Read the model definition and answer for the solid it produces. Units are mm, in the model's axes. A direction names the side the tool comes from. Coordinates: 2 decimals unless noted, no trailing zeros. Order: outer loops, then holes, each group sorted by start corner. A loop starts at its lowest first (then second) coordinate and runs counter-clockwise, first axis right, second up. Notation, with made-up numbers: (-25, -16) -> (-13, -16) arc R20 ccw to (-13, 3) -> close; hole circle Ø10 at (87.25, 28). An arc over 180 degrees is marked (long way). Use CSV: the item, a comma, the result in double quotes.
```python
from build123d import *

# Parameters (mm, degrees)
F1_DEPTH = 80
F2_R     = 7.5
F3_DEPTH = 40
F4_R     = 2.5
F5_DEPTH = 50


with BuildPart() as f1:
    # F0 (on Front) → F1 (new body)
    with BuildSketch(Plane.XZ):
        Polygon((13.916367, 60.022387), (-11.083633, 60.022387), (-11.083633, -19.977613), (-6.383633, -19.977613), (-6.383633, 40.022387), (9.216367, 40.022387), (9.216367, -19.977613), (13.916367, -19.977613), align=None)
    extrude(amount=F1_DEPTH)

    # F2 (on face) → F3 (join)
    with BuildSketch(Plane.XY.offset(60.022387)):
        with Locations((1.416367, -40)):
            Circle(F2_R)
    extrude(amount=F3_DEPTH)

    # F4 (on face) → F5 (cut)
    with BuildSketch(Plane.YZ.offset(13.916367)):
        with Locations((-62.5, -2.477613)):
            Circle(F4_R)
        with Locations((-17.5, -2.477613)):
            Circle(F4_R)
    extrude(amount=-F5_DEPTH, mode=Mode.SUBTRACT)


solid = f1.part
```
Item 1: Find section D-D, the plane x = 11. Give the vertices of the cut face in (y, z).
Return value:
outline,"(-80, -19.98) -> (0, -19.98) -> (0, 60.02) -> (-80, 60.02) -> close; hole circle Ø5 at (-62.5, -2.48); hole circle Ø5 at (-17.5, -2.48)"
Item 2: Find section C-C, the plane y = -40. Give the vertices of the cut face in (x, z).
Return value:
outline,"(-11.08, -19.98) -> (-6.38, -19.98) -> (-6.38, 40.02) -> (9.22, 40.02) -> (9.22, -19.98) -> (13.92, -19.98) -> (13.92, 60.02) -> (8.92, 60.02) -> (8.92, 100.02) -> (-6.08, 100.02) -> (-6.08, 60.02) -> (-11.08, 60.02) -> close"
Item 3: The mould has two halves that part along Y. Classify faces 1 (the flat face through (9.216, -39, 10)), 2 (the cylindrical face through (-0.21, -47.32, 79.74)), 3 (the cylindrical face through (-8.7, -20, -2.4)): +Y half, -Y half, draft (parallel to the pull), parting line (faces both ways), or undercut.
Return value:
face 1,"draft"
face 2,"parting line"
face 3,"undercut"
Item 4: Find section B-B, the plane y = -62.5. Give the vertices of the cut face in (x, z).
Return value:
outline,"(-11.08, -19.98) -> (-6.38, -19.98) -> (-6.38, -4.98) -> (-11.08, -4.98) -> close; (-11.08, 0.02) -> (-6.38, 0.02) -> (-6.38, 40.02) -> (9.22, 40.02) -> (9.22, 0.02) -> (13.92, 0.02) -> (13.92, 60.02) -> (-11.08, 60.02) -> close; (9.22, -19.98) -> (13.92, -19.98) -> (13.92, -4.98) -> (9.22, -4.98) -> close"
Item 5: Straight lines are drawn through the part: line 1 along Z through (x, y) = (10.3, -17.5); line 2 along X through (y, z) = (-23, 28); line 3 along Z through (x, y) = (0.25, -39). For each, find the intervals that lie inside material, in ascending order.
Return value:
line 1,"z = -19.98 to -4.98, 0.02 to 60.02"
line 2,"x = -11.08 to -6.38, 9.22 to 13.92"
line 3,"z = 40.02 to 100.02"
Item 6: Find section A-A, the plane z = -11. Give the vertices of the cut face in (x, y), then the cut area to 3 significant figures.
Return value:
outline,"(-11.08, -80) -> (-6.38, -80) -> (-6.38, 0) -> (-11.08, 0) -> close; (9.22, -80) -> (13.92, -80) -> (13.92, 0) -> (9.22, 0) -> close"
area,"752 mm^2"
Item 7: Each of these flat-tipped pins is pushed along its axis until it touches: P1, Ø5, axis at x = 2, y = -8.5, coming from the -Z side; P2, Ø4, axis at x = 3, z = 85, coming from the -Y side; P3, Ø1, axis at x = -3.5, y = -32, coming from the +Z side. Where does it stop, or does it pass through?
Return value:
P1,"stops at z = 40.02"
P2,"stops at y = -47.5"
P3,"stops at z = 60.02"
Item 8: A tool of negligible diameter and unlimited length cuts with its end or side. For faces 4 (the cylindrical face through (11.6, -20, -2.4)), 5 (the flat face through (-6.384, -39, 10)), from which of +Z, -Z, +X, -X, +Y, -Y can it reach the whole face along a straight path? Write none if from no direction.
Return value:
face 4,"+X, -X"
face 5,"-Z, +Y, -Y"
